Print and shaded views of the part. All mm, measured from the part's lowest x, y and z. Give positions to 0.01 mm unless a question says otherwise; leave off trailing zeros. Loops run counter-clockwise (first coordinate to the right, second up) from the corner with the lowest first, then second, coordinate; pieces in that order, holes last. Notation, with made-up numbers: M 19,41 L 52,41 A15 ccw 52,50 Z; hole C 30,1.25 d8. An arc over 180 degrees is marked long. Answer in a Markdown table with one row per item.
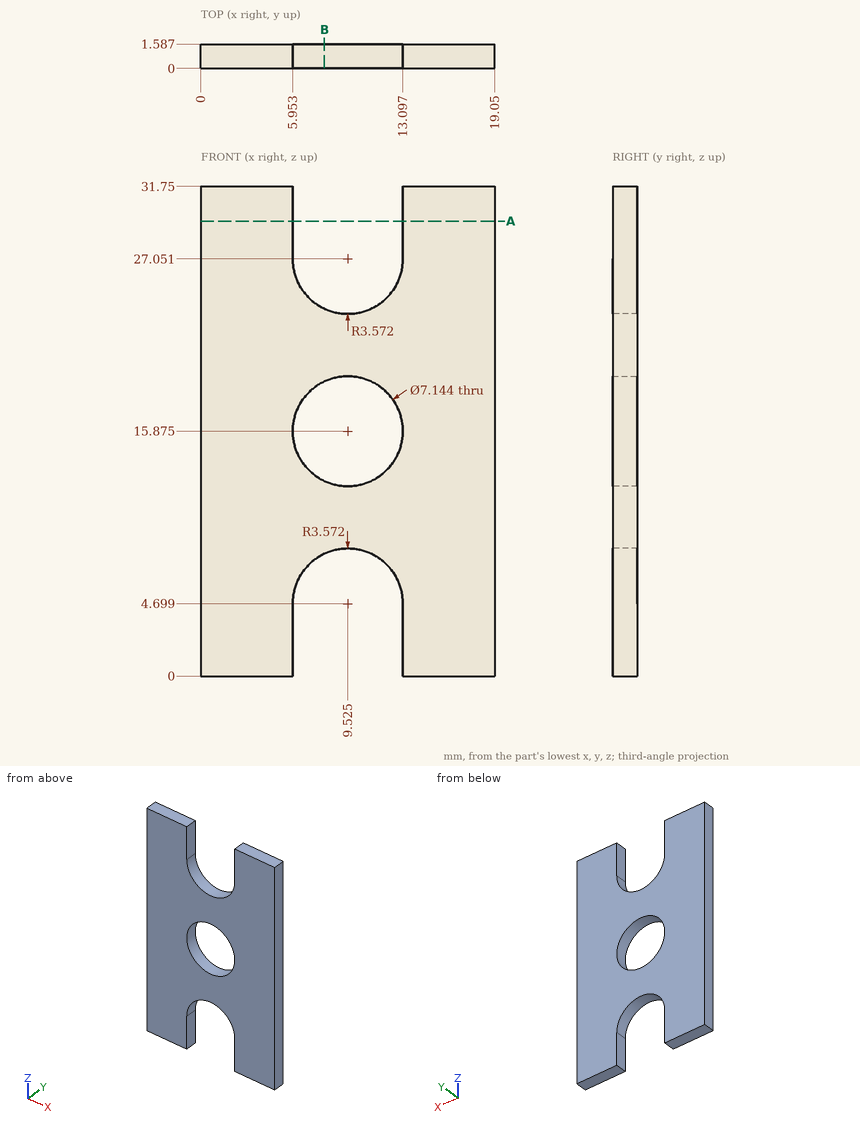
(1) Flat gauge pin, fed straight in: P1, Ø5.5, axis at x = 9.525, z = 15.875, coming from the +Y side. Where does the tip first touch, or does it go through?
Established:
| item | result |
|---|---|
| P1 | passes through |
(2) Wall check: L1, parallel to X at y = 0.2, z = 27.5; L2, parallel to Z at x = 9.5, y = 0.35; L3, parallel to Z at x = 12.25, y = 1.4 (1 decimal). Give the ranges that are in metal, low to high.
Established:
| item | result |
|---|---|
| L1 | x = 0 to 5.95, 13.1 to 19.05 |
| L2 | z = 8.27 to 12.3, 19.45 to 23.48 |
| L3 | z = 7 to 13.6, 18.2 to 24.7 |
(3) Saw through at A-A, the plane z = 29.5. Give the cut face in (x, y).
Established:
| item | result |
|---|---|
| outline | M 0,0 L 5.95,0 L 5.95,1.59 L 0,1.59 Z; M 13.1,0 L 19.05,0 L 19.05,1.59 L 13.1,1.59 Z |
(4) Saw through at B-B, the plane x = 8. Give the cut face in (y, z) (1 decimal).
Established:
| item | result |
|---|---|
| outline | M 0,7.9 L 1.6,7.9 L 1.6,12.6 L 0,12.6 Z; M 0,19.1 L 1.6,19.1 L 1.6,23.8 L 0,23.8 Z |
